Print and shaded views of the part. All mm, measured from the part's lowest x, y and z. Round coordinates to 2 decimals unless told otherwise and drop trailing zeros. Write each loop counter-clockwise with the first axis right and the second up, starting at its lowest first coordinate (ties: lowest second). Pieces come first, ordered by that corner, then holes. Notation, with made-up numbers: (55.25, 18) -> (87.25, 18) arc R11 cw to (87.25, 22) -> close; hole circle Ø6 at (-38, -22). An arc over 180 degrees is marked (long way). Use CSV: the item, a comma, the result in double quotes. Start each with the question number.
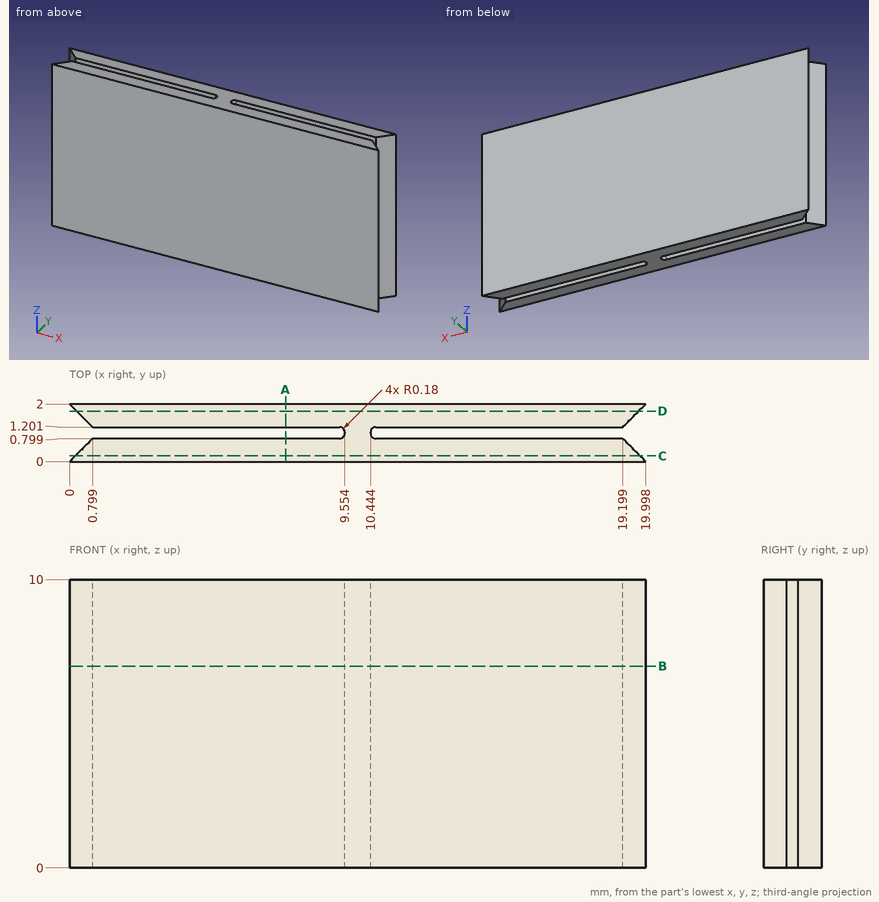
1. Band-saw the part on A-A (x = 7.5). List the corners of the cut face in (y, z).
2. Band-saw the part on B-B (z = 7). List the corners of the cut face in (x, y).
3. Band-saw the part on C-C (y = 0.2). List the corners of the cut face in (x, z).
4. Drill centre lines: line 1 along Y through (x, z) = (19, 7.5); line 2 along X through (y, z) = (1, 4.75); line 3 along X through (y, z) = (0.5, 9) (1 decimal). Where is each one in solid material? Low to high. Write a range as [from, to].
5. Band-saw the part on D-D (y = 1.75). List the corners of the cut face in (x, z).
Answers below:
1,outline,"(0, 0) -> (0.8, 0) -> (0.8, 10) -> (0, 10) -> close; (1.2, 0) -> (2, 0) -> (2, 10) -> (1.2, 10) -> close"
2,outline,"(0, 0) -> (20, 0) -> (19.2, 0.8) -> (10.62, 0.8) arc R0.18 cw to (10.44, 0.98) -> (10.44, 1.02) arc R0.18 cw to (10.62, 1.2) -> (19.2, 1.2) -> (20, 2) -> (0, 2) -> (0.8, 1.2) -> (9.37, 1.2) arc R0.18 cw to (9.55, 1.02) -> (9.55, 0.98) arc R0.18 cw to (9.37, 0.8) -> (0.8, 0.8) -> close"
3,outline,"(0.2, 0) -> (19.8, 0) -> (19.8, 10) -> (0.2, 10) -> close"
4,line 1,"y = [0, 0.8], [1.2, 2]"
4,line 2,"x = [9.55, 10.44]"
4,line 3,"x = [0.5, 19.5]"
5,outline,"(0.25, 0) -> (19.75, 0) -> (19.75, 10) -> (0.25, 10) -> close"
